Answer from the drawing. Dimensions are ordinates in mm from the lowest x, y and z of the part. Coordinates: 2 decimals unless noted, no trailing zeros. Write each loop counter-clockwise with the first axis right and the second up, starting at its lowest first coordinate (ties: lowest second). Pieces come first, ordered by that corner, then holes.
(1) Given P1, Ø0.5, axis at x = 7.5, z = 0.5, coming from the -Y side, flat-ended and moving along its own axis, determine where the tip first touches the part or whether it passes through.
(2) Straight lines are drawn through the part: line 1 (Y direction, x = 25, z = 0.55); line 2 (X direction, y = 35.5, z = 0.8); line 3 (Y direction, x = 5, z = 0.7). For each, find the intervals that lie inside material, in ascending order.
(3) The part is cut by section D-D on x = 25. Determine the outline of the cut face in (y, z).
(4) The part is cut by section C-C on z = 0.25. Give the number of separate pieces and of enclosed holes in the cut face, plus the area to 3 significant figures.
(5) The part is cut by section B-B on x = 15. Determine the outline of the cut face in (y, z).
(6) The part is cut by section A-A on y = 5. Determine the outline of the cut face in (x, z).
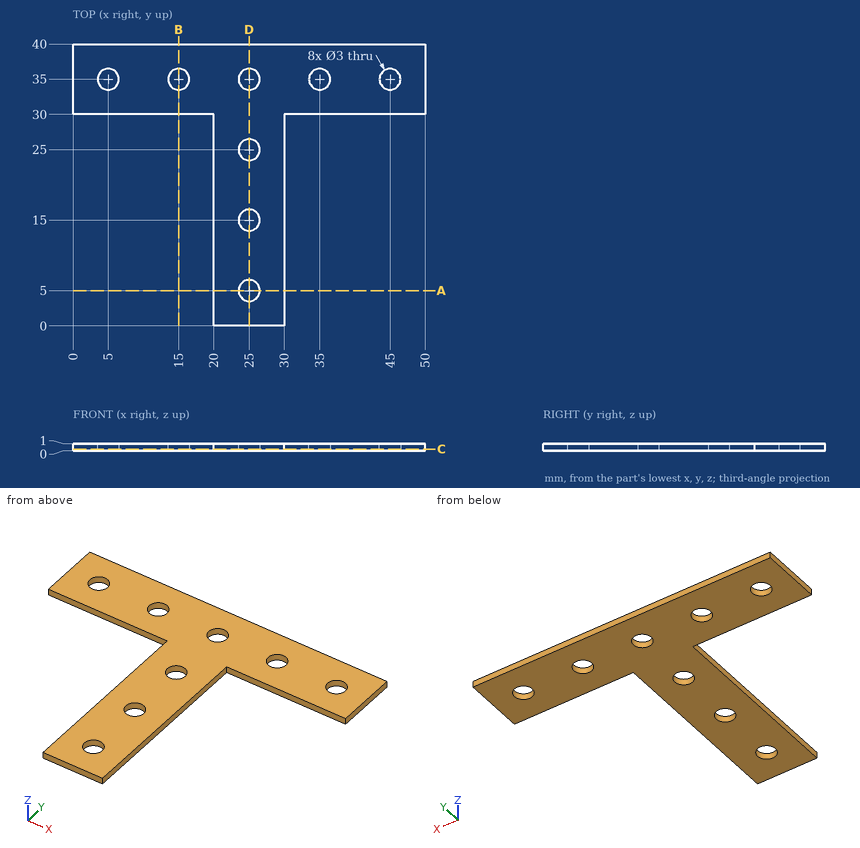
Model answer:
1. P1: stops at y = 30
2. line 1: y = 0 to 3.5, 6.5 to 13.5, 16.5 to 23.5, 26.5 to 33.5, 36.5 to 40
2. line 2: x = 0 to 3.59, 6.41 to 13.59, 16.41 to 23.59, 26.41 to 33.59, 36.41 to 43.59, 46.41 to 50
2. line 3: y = 30 to 33.5, 36.5 to 40
3. outline: (0, 0) - (3.5, 0) - (3.5, 1) - (0, 1) - close; (6.5, 0) - (13.5, 0) - (13.5, 1) - (6.5, 1) - close; (16.5, 0) - (23.5, 0) - (23.5, 1) - (16.5, 1) - close; (26.5, 0) - (33.5, 0) - (33.5, 1) - (26.5, 1) - close; (36.5, 0) - (40, 0) - (40, 1) - (36.5, 1) - close
4. separate pieces: 1
4. enclosed holes: 8
4. area: 743 mm2
5. outline: (30, 0) - (33.5, 0) - (33.5, 1) - (30, 1) - close; (36.5, 0) - (40, 0) - (40, 1) - (36.5, 1) - close
6. outline: (20, 0) - (23.5, 0) - (23.5, 1) - (20, 1) - close; (26.5, 0) - (30, 0) - (30, 1) - (26.5, 1) - close
